For this review, take the finished solid that the model builds, in its own axes (mm). Give positions to 0.01 mm unless a question says otherwise; leave off trailing zeros. Write each loop counter-clockwise with the first axis right and the second up, starting at its lowest first coordinate (ties: lowest second). Pieces come first, ordered by that corner, then holes. Notation, with made-up numbers: M -22.5,73 L -14.5,73 A21 ccw -14.5,96 Z; hole C 61,-4 d8. An arc over 180 degrees is marked long. Answer as a JSON object with one key per item and string values. Group by question number.
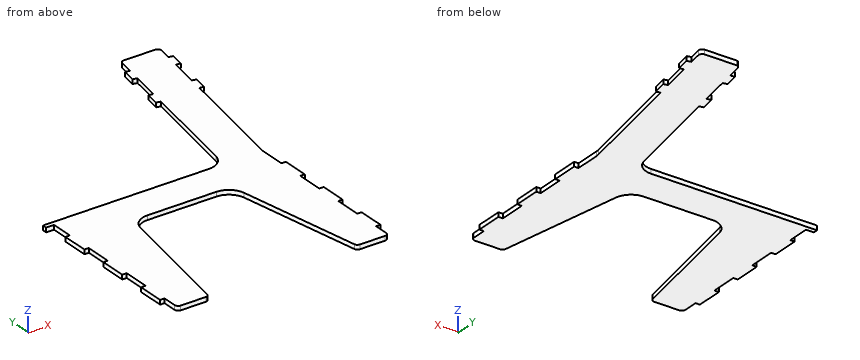
```python
from build123d import *

# Parameters (mm, degrees)
BOSS_EXTRUDE1_DEPTH = 2.5
FILLET1_R           = 2
FILLET2_R           = 10


with BuildPart() as part:
    # Sketch1 → Boss-Extrude1 (new body)
    with BuildSketch(Plane.XY):
        Polygon((-42, -90), (-27.893841543, -10), (27.893841543, -10), (42, -90), (60, -90), (60, -80), (62.5, -80), (62.5, -65), (60, -65), (60, -50), (62.5, -50), (62.5, -35), (60, -35), (60, -20), (62.5, -20), (62.5, -5), (60, -5), (60, 10), (71.710975051, 76.416239896), (74.172994433, 75.982119452), (75.562179855, 83.860581476), (73.100160472, 84.29470192), (76.052179493, 101.036433721), (78.514198875, 100.602313277), (79.903384296, 108.480775301), (77.441364914, 108.914895745), (79.101299543, 118.328852831), (57.068895795, 118.328852831), (55.332414019, 108.480775301), (52.870394636, 108.914895745), (51.481209215, 101.036433721), (53.943228597, 100.602313277), (50.991209577, 83.860581476), (48.529190194, 84.29470192), (47.140004773, 76.416239896), (49.602024156, 75.982119452), (37.967596252, 10), (-64.5, 10), (-64.5, 7.5), (-60, 7.5), (-60, -5), (-62.5, -5), (-62.5, -20), (-60, -20), (-60, -35), (-62.5, -35), (-62.5, -50), (-60, -50), (-60, -65), (-62.5, -65), (-62.5, -80), (-60, -80), (-60, -90), align=None)
    extrude(amount=BOSS_EXTRUDE1_DEPTH)

    # Fillet1
    fillet1_edges = [part.edges().sort_by_distance(p)[0] for p in [
        (60, -90, 1.25),
        (42, -90, 1.25),
        (-42, -90, 1.25),
        (-60, -90, 1.25),
        (57.068895795, 118.328852831, 1.25),
        (79.101299543, 118.328852831, 1.25),
    ]]
    fillet(fillet1_edges, radius=FILLET1_R)

    # Fillet2
    fillet2_edges = [part.edges().sort_by_distance(p)[0] for p in [
        (27.893841543, -10, 1.25),
        (-27.893841543, -10, 1.25),
        (37.967596252, 10, 1.25),
        (60, 10, 1.25),
    ]]
    fillet(fillet2_edges, radius=FILLET2_R)


solid = part.part
```
Item 1: Consider section A-A (y = -27). Give the boundary of the cut face in (x, z), plus the area to 3 significant figures.
Item 2: Consider section C-C (y = 68). Give the boundary of the cut face in (x, z).
Item 3: Insertion check: P1, Ø0.8, axis at y = -45.5, z = 1, coming from the +X side; P2, Ø0.8, axis at y = -83, z = 1, coming from the +X side; P3, Ø1.2, axis at x = -61, z = 2, coming from the +Y side. Each pin has a flat end and moves straight along its axis. Give the tip position at first contact, or say it passes through.
Item 4: Consider section B-B (x = 16.5). Give the boundary of the cut face in (y, z), plus the area to 3 significant figures.
Item 5: To check wall thickness, follow probe 1 along Y at (x, z) = (-13.5, 0.3); probe 2 along Y at (x, z) = (-52, 1.15); probe 3 along X at (y, z) = (-77, 1.6). State the ranges of each line that lie inside material, in increasing order.
Result set:
{
 "1": {"outline": "M -60,0 L -30.89,0 L -30.89,2.5 L -60,2.5 Z; M 30.89,0 L 60,0 L 60,2.5 L 30.89,2.5 Z", "area": "146 mm^2"},
 "2": {"outline": "M 48.19,0 L 70.23,0 L 70.23,2.5 L 48.19,2.5 Z"},
 "3": {"P1": "stops at x = 62.5", "P2": "stops at x = 60", "P3": "stops at y = 10"},
 "4": {"outline": "M -10,0 L 10,0 L 10,2.5 L -10,2.5 Z", "area": "50.0 mm^2"},
 "5": {"probe 1": "y = -10 to 10", "probe 2": "y = -90 to 10", "probe 3": "x = -62.5 to -39.71, 39.71 to 62.5"}
}
